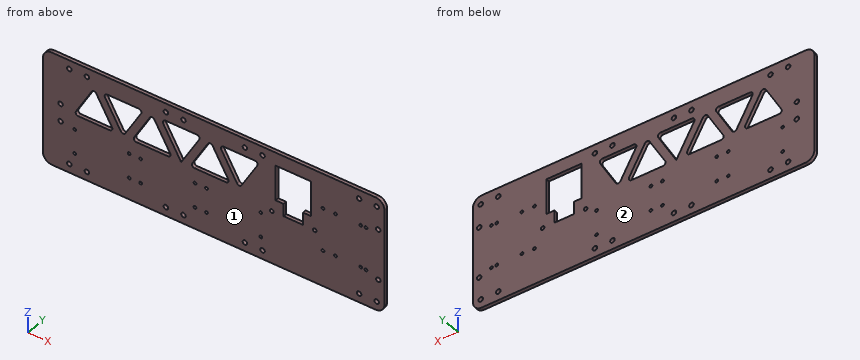
```python
from build123d import *

# Parameters (mm, degrees)
SKETCH_1_W          = 388.85
SKETCH_1_H          = 130
EXTRUDE_1_DEPTH     = 4
SKETCH_2_R          = 1.6
CUT_EXTRUDE_1_DEPTH = 4
SKETCH_3_R          = 2.6
CUT_EXTRUDE_2_DEPTH = 411.024782788
SKETCH_5_R          = 2.6
CUT_EXTRUDE_3_DEPTH = 411.024782788
SKETCH_7_R          = 2.1
CUT_EXTRUDE_5_DEPTH = 411.024782788
SKETCH_8_R          = 1.6
CUT_EXTRUDE_6_DEPTH = 411.024782788
SKETCH_9_R          = 1.6
CUT_EXTRUDE_7_DEPTH = 411.024782788
SKETCH_10_R         = 2.6
CUT_EXTRUDE_8_DEPTH = 411.024782788
FILLET_1_R          = 10
CUT_EXTRUDE_9_DEPTH = 411.024782788
FILLET_2_R          = 3


with BuildPart() as part:
    # 草图1 → 凸台-拉伸1 (new body)
    with BuildSketch(Plane(origin=(0, 0, 0), x_dir=(1, 0, 0), z_dir=(0, 1, 0))):
        with Locations((194.425, -65)):
            Rectangle(SKETCH_1_W, SKETCH_1_H)
    extrude(amount=EXTRUDE_1_DEPTH)

    # 草图2 → 切除-拉伸1 (cut)
    with BuildSketch(Plane(origin=(0, 4, 0), x_dir=(1, 0, 0), z_dir=(0, 1, 0))):
        with Locations(Location((36.21, -52.9, 0), (0, 0, 270))):
            Circle(SKETCH_2_R)
        with Locations(Location((98.11, -52.9, 0), (0, 0, 270))):
            Circle(SKETCH_2_R)
        with Locations(Location((98.11, -24.8, 0), (0, 0, 270))):
            Circle(SKETCH_2_R)
        with Locations(Location((111.21, -24.8, 0), (0, 0, 270))):
            Circle(SKETCH_2_R)
        with Locations(Location((111.21, -52.9, 0), (0, 0, 270))):
            Circle(SKETCH_2_R)
        with Locations(Location((173.11, -24.8, 0), (0, 0, 270))):
            Circle(SKETCH_2_R)
        with Locations(Location((173.11, -52.9, 0), (0, 0, 270))):
            Circle(SKETCH_2_R)
        with Locations(Location((186.21, -24.8, 0), (0, 0, 270))):
            Circle(SKETCH_2_R)
        with Locations(Location((186.21, -52.9, 0), (0, 0, 270))):
            Circle(SKETCH_2_R)
        with Locations(Location((248.11, -52.9, 0), (0, 0, 270))):
            Circle(SKETCH_2_R)
        with Locations(Location((36.21, -24.8, 0), (0, 0, 270))):
            Circle(SKETCH_2_R)
        with Locations(Location((248.11, -24.8, 0), (0, 0, 270))):
            Circle(SKETCH_2_R)
    extrude(amount=-CUT_EXTRUDE_1_DEPTH, mode=Mode.SUBTRACT)

    # 草图3 → 切除-拉伸2 (cut, through all)
    with BuildSketch(Plane(origin=(0, 4, 0), x_dir=(1, 0, 0), z_dir=(0, 1, 0))):
        with Locations(Location((20, -75, 0), (0, 0, 270))):
            Circle(SKETCH_3_R)
        with Locations(Location((20, -55, 0), (0, 0, 270))):
            Circle(SKETCH_3_R)
    extrude(amount=-CUT_EXTRUDE_2_DEPTH, mode=Mode.SUBTRACT)

    # 草图5 → 切除-拉伸3 (cut, through all)
    with BuildSketch(Plane(origin=(0, 4, 0), x_dir=(1, 0, 0), z_dir=(0, 1, 0))):
        with Locations(Location((30, -10, 0), (0, 0, 270))):
            Circle(SKETCH_5_R)
        with Locations(Location((50, -10, 0), (0, 0, 270))):
            Circle(SKETCH_5_R)
        with Locations(Location((140, -10, 0), (0, 0, 270))):
            Circle(SKETCH_5_R)
        with Locations(Location((160, -10, 0), (0, 0, 270))):
            Circle(SKETCH_5_R)
        with Locations(Location((230, -10, 0), (0, 0, 270))):
            Circle(SKETCH_5_R)
        with Locations(Location((250, -10, 0), (0, 0, 270))):
            Circle(SKETCH_5_R)
        with Locations(Location((360, -10, 0), (0, 0, 270))):
            Circle(SKETCH_5_R)
        with Locations(Location((380, -10, 0), (0, 0, 270))):
            Circle(SKETCH_5_R)
        with Locations(Location((380, -120, 0), (0, 0, 90))):
            Circle(SKETCH_5_R)
        with Locations(Location((360, -120, 0), (0, 0, 90))):
            Circle(SKETCH_5_R)
        with Locations(Location((250, -120, 0), (0, 0, 90))):
            Circle(SKETCH_5_R)
        with Locations(Location((230, -120, 0), (0, 0, 90))):
            Circle(SKETCH_5_R)
        with Locations(Location((160, -120, 0), (0, 0, 90))):
            Circle(SKETCH_5_R)
        with Locations(Location((140, -120, 0), (0, 0, 90))):
            Circle(SKETCH_5_R)
        with Locations(Location((50, -120, 0), (0, 0, 90))):
            Circle(SKETCH_5_R)
        with Locations(Location((30, -120, 0), (0, 0, 90))):
            Circle(SKETCH_5_R)
    extrude(amount=-CUT_EXTRUDE_3_DEPTH, mode=Mode.SUBTRACT)

    # 草图7 → 切除-拉伸5 (cut, through all)
    with BuildSketch(Plane(origin=(0, 4, 0), x_dir=(1, 0, 0), z_dir=(0, 1, 0))):
        with Locations(Location((260.6, -60.4, 0), (0, 0, 270))):
            Circle(SKETCH_7_R)
        with Locations(Location((309.6, -60.4, 0), (0, 0, 90))):
            Circle(SKETCH_7_R)
        Polygon((305.2, -74.8), (305.2, -115), (265, -115), (265, -74.8), (274.1, -74.8), (274.1, -60.5), (296.1, -60.5), (296.1, -74.8), align=None)
    extrude(amount=-CUT_EXTRUDE_5_DEPTH, mode=Mode.SUBTRACT)

    # 草图8 → 切除-拉伸6 (cut, through all)
    with BuildSketch(Plane(origin=(0, 4, 0), x_dir=(1, 0, 0), z_dir=(0, 1, 0))):
        with Locations(Location((318.85, -41, 0), (0, 0, 270))):
            Circle(SKETCH_8_R)
        with Locations(Location((367.85, -41, 0), (0, 0, 270))):
            Circle(SKETCH_8_R)
        with Locations(Location((318.85, -90, 0), (0, 0, 270))):
            Circle(SKETCH_8_R)
        with Locations(Location((367.85, -90, 0), (0, 0, 270))):
            Circle(SKETCH_8_R)
    extrude(amount=-CUT_EXTRUDE_6_DEPTH, mode=Mode.SUBTRACT)

    # 草图9 → 切除-拉伸7 (cut, through all)
    with BuildSketch(Plane(origin=(0, 4, 0), x_dir=(1, 0, 0), z_dir=(0, 1, 0))):
        with Locations(Location((333.15, -41.5, 0), (0, 0, 270))):
            Circle(SKETCH_9_R)
        with Locations(Location((361.85, -41.5, 0), (0, 0, 270))):
            Circle(SKETCH_9_R)
        with Locations(Location((333.15, -90, 0), (0, 0, 270))):
            Circle(SKETCH_9_R)
        with Locations(Location((361.85, -90, 0), (0, 0, 270))):
            Circle(SKETCH_9_R)
    extrude(amount=-CUT_EXTRUDE_7_DEPTH, mode=Mode.SUBTRACT)

    # 草图10 → 切除-拉伸8 (cut, through all)
    with BuildSketch(Plane(origin=(0, 4, 0), x_dir=(1, 0, 0), z_dir=(0, 1, 0))):
        with Locations(Location((381.85, -36, 0), (0, 0, 270))):
            Circle(SKETCH_10_R)
        with Locations(Location((381.85, -94, 0), (0, 0, 90))):
            Circle(SKETCH_10_R)
    extrude(amount=-CUT_EXTRUDE_8_DEPTH, mode=Mode.SUBTRACT)

    # 圆角1
    fillet_1_edges = [part.edges().sort_by_distance(p)[0] for p in [
        (0, 2, 0),
        (388.85, 2, 0),
        (388.85, 2, 130),
        (0, 2, 130),
    ]]
    fillet(fillet_1_edges, radius=FILLET_1_R)

    # 草图11 → 切除-拉伸9 (cut, through all)
    with BuildSketch(Plane(origin=(0, 4, 0), x_dir=(1, 0, 0), z_dir=(0, 1, 0))):
        Polygon((58.095, -110.001713401), (81.19, -70), (35, -70), align=None)
        Polygon((68.095, -110.001713401), (114.285, -110.001713401), (91.19, -70), align=None)
        Polygon((124.285, -110.001713401), (147.38, -70), (101.19, -70), align=None)
        Polygon((134.285, -110.001713401), (180.475, -110.001713401), (157.38, -70), align=None)
        Polygon((190.475, -110.001713401), (213.57, -70), (167.38, -70), align=None)
        Polygon((200.475, -110.001713401), (246.665, -110.001713401), (223.57, -70), align=None)
    extrude(amount=-CUT_EXTRUDE_9_DEPTH, mode=Mode.SUBTRACT)

    # 圆角2
    fillet_2_edges = [part.edges().sort_by_distance(p)[0] for p in [
        (134.285, 2, 110.001713401),
        (180.475, 2, 110.001713401),
        (190.475, 2, 110.001713401),
        (167.38, 2, 70),
        (213.57, 2, 70),
        (68.095, 2, 110.001713401),
        (91.19, 2, 70),
        (114.285, 2, 110.001713401),
        (124.285, 2, 110.001713401),
        (101.19, 2, 70),
        (147.38, 2, 70),
        (200.475, 2, 110.001713401),
        (223.57, 2, 70),
        (246.665, 2, 110.001713401),
        (58.095, 2, 110.001713401),
        (35, 2, 70),
        (81.19, 2, 70),
    ]]
    fillet(fillet_2_edges, radius=FILLET_2_R)


solid = part.part
```
Check sheet for the modelled part. Datum: model origin and axes. Units: mm. Face numbers are marked on the shaded views. Round coordinates to 2 decimals unless told otherwise and drop trailing zeros. One line per question, with ' | ' between items. Start each with the question number.
1. Depth check by flat-ended pin: pin 1 (10 mm diameter, centred on x = 345, z = 69.5, fed in from -Y). Enter the tip coordinate at first touch or a pass-through.
2. Release check for a two-part mould opening along Y. For the marked faces 1 and 2 record: +Y half, -Y half, draft (parallel to the pull), parting line (faces both ways), or undercut.
3. Sectioned sample at A-A, the plane y = 1.05. Count the separate pieces of the cut face and the enclosed holes in it, then the cut area to 3 significant figures.
4. Scan lines: line 1 along Z through (x, y) = (160, 2.95); line 2 along Z through (x, y) = (250, 1.5); line 3 along Z through (x, y) = (19.5, 3.75). Record each from-to range of solid material in increasing order. Write a range as from..to.
Taken from the geometry:
1) pin 1: stops at y = 0
2) face 1: -Y half | face 2: +Y half
3) separate pieces: 1 | enclosed holes: 49 | area: 42,500 mm^2
4) line 1: z = 0..7.4, 12.6..74.54, 110..117.4, 122.6..130 | line 2: z = 0..7.4, 12.6..117.4, 122.6..130 | line 3: z = 0..52.45, 57.55..72.45, 77.55..130
